The drawing under review shows one solid part. Ordinate dimensions are in mm from its lowest x, y, z. Give positions to 0.01 mm unless a question says otherwise; leave off trailing zeros. Write each loop counter-clockwise with the first axis right and the second up, starting at its lowest first coordinate (ties: lowest second). Pieces come first, ordered by that corner, then holes. Notation, with made-up numbers: (83, 14) -> (106, 14) arc R14 cw to (106, 38) -> close; hole circle Ø9 at (88, 27). An arc over 180 degrees is marked (long way). Write item = value, one per line.
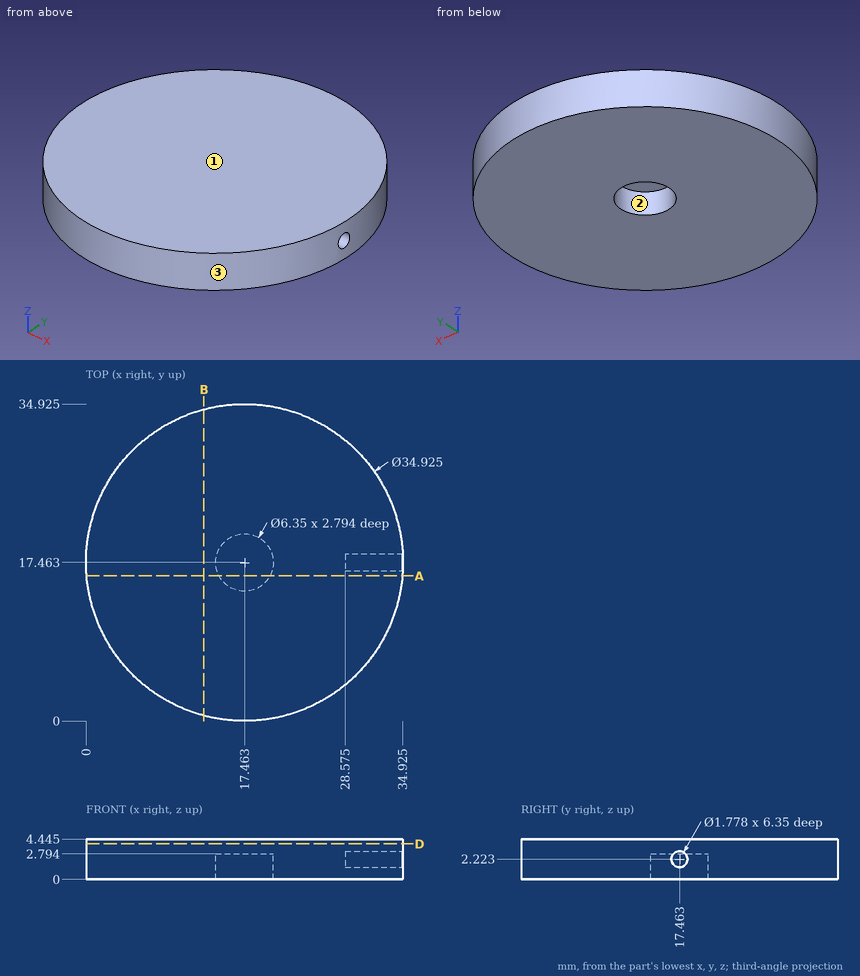
(1) Take a section at D-D (z = 3.9). Write out the cut boundary in (x, y) (1 decimal).
Answers below:
outline = circle Ø34.9 at (17.5, 17.5)
(2) Take a section at A-A (y = 16). Write out the cut boundary in (x, z) (1 decimal), plus the area to 3 significant figures.
Answers below:
outline = (0.1, 0) -> (14.6, 0) -> (14.6, 2.8) -> (20.3, 2.8) -> (20.3, 0) -> (34.9, 0) -> (34.9, 4.4) -> (0.1, 4.4) -> close
area = 139 mm^2
(3) The part is to be moulded in two halves that separate along X. For the marked faces 1, 2 and 3, say which applies: released by +X, released by -X, zero draft, split by the parting line, or undercut.
Answers below:
face_1 = zero draft
face_2 = undercut
face_3 = split by the parting line
(4) To check wall thickness, follow probe 1 along Y at (x, z) = (16, 0.6) (1 decimal); probe 2 along Z at (x, y) = (16, 20) (1 decimal); probe 3 along X at (y, z) = (16.5, 1.25) (1 decimal). State the ranges of each line that lie inside material, in increasing order.
Answers below:
probe_1 = 0.1 to 14.6, 20.3 to 34.9
probe_2 = 2.8 to 4.4
probe_3 = 0 to 14.4, 20.5 to 34.9
(5) For pin 1 (1.5 mm diameter, centred on y = 15.5, z = 3, fed in from -X); pin 2 (3 mm diameter, centred on x = 18.5, y = 19, fed in from -Z); pin 3 (1.5 mm diameter, centred on x = 5, z = 3, fed in from -Y); pin 4 (1.5 mm diameter, centred on y = 10.5, z = 2, fed in from -X), all flat-tipped, find the tip position at first contact; note any pin that passes through.
Answers below:
pin_1 = 0.04
pin_2 = 0
pin_3 = 4.51
pin_4 = 1.14
(6) Take a section at B-B (x = 13). Write out the cut boundary in (y, z) (1 decimal), plus the area to 3 significant figures.
Answers below:
outline = (0.6, 0) -> (34.3, 0) -> (34.3, 4.4) -> (0.6, 4.4) -> close
area = 150 mm^2
